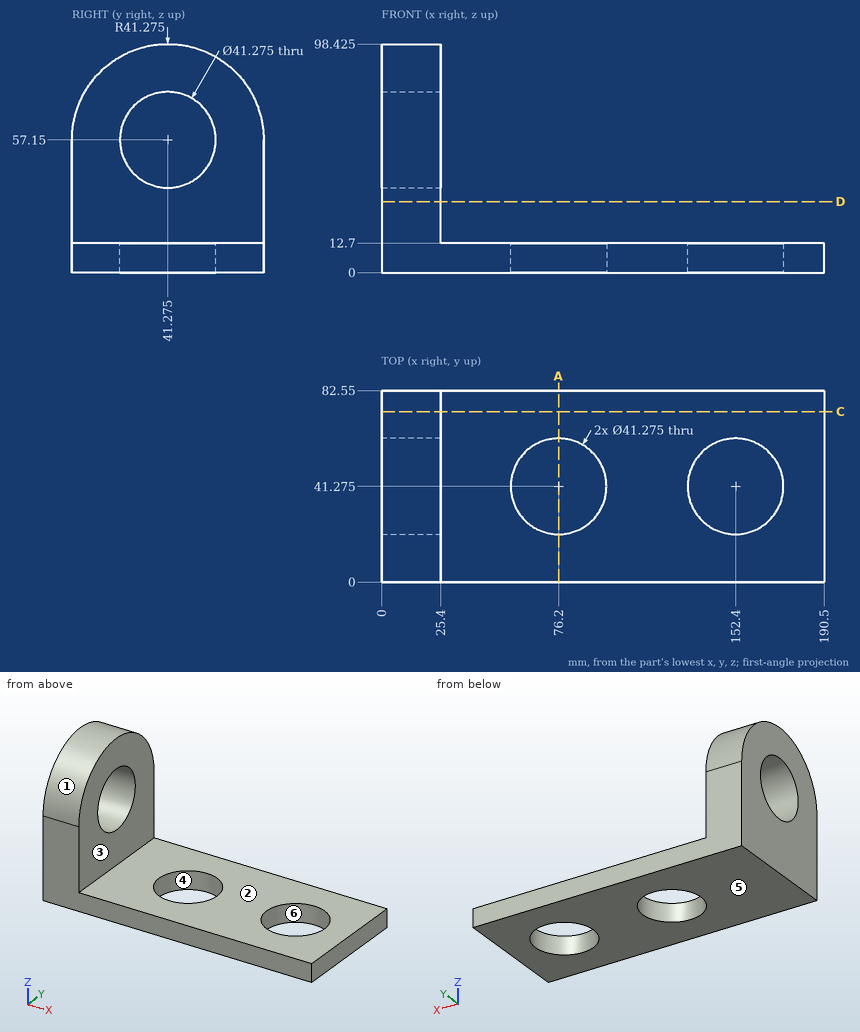
For this review, use the dimensioned drawing (mm, ordinates from the lowest corner) and the shaded views. A direction names the side the tool comes from. Round coordinates to 2 decimals unless told otherwise and drop trailing zeros. Order: outer loops, then holes, each group sorted by start corner. A loop starts at its lowest first (then second) coordinate and runs counter-clockwise, first axis right, second up. Notation, with made-up numbers: (-6, 67) -> (17, 67) arc R24 cw to (17, 90) -> close; hole circle Ø5 at (-4, 74.25). An arc over 180 degrees is marked (long way). Put each result on its own line as item: value.
Q1. Add section A-A on x = 76.2. Write out the cut boundary in (y, z).
Check result:
outline: (0, 0) -> (20.64, 0) -> (20.64, 12.7) -> (0, 12.7) -> close; (61.91, 0) -> (82.55, 0) -> (82.55, 12.7) -> (61.91, 12.7) -> close
Q2. Add section C-C on y = 73.5. Write out the cut boundary in (x, z), plus the area to 3 significant figures.
Check result:
outline: (0, 0) -> (190.5, 0) -> (190.5, 12.7) -> (25.4, 12.7) -> (25.4, 82.94) -> (0, 82.94) -> close
area: 4,200 mm2
Q3. Insertion check: pin 1 Ø4 at (y, z) = (34, 25.5) entering from +X. The pin has a flat end and moves straight along its axis. Give the tip position at first contact, or say it passes through.
Check result:
pin 1: x = 25.4
Q4. Mouldability with a two-part tool opening along X and no side actions: class the marked faces 3, 4, 5 and 6 as pulls with the +X half, pulls with the -X half, needs draft (parallel to the pull), parting line crosses it, or undercut.
Check result:
face 3: pulls with the +X half
face 4: undercut
face 5: needs draft
face 6: undercut
Q5. Machinability: for the marked faces 1 and 2, which of the approach directions +Z, -Z, +X, -X, +Y, -Y give a long, thin tool a straight path to every point of the face, cutting with its end or side? Answer none if there is none.
Check result:
face 1: +Z, +X, -X
face 2: +Z, +X, +Y, -Y
Q6. Add section D-D on z = 30.5. Write out the cut boundary in (x, y), plus the area to 3 significant figures.
Check result:
outline: (0, 0) -> (25.4, 0) -> (25.4, 82.55) -> (0, 82.55) -> close
area: 2,100 mm2
Q7. For probe 1 along Y at (x, z) = (152.4, 9.5); probe 2 along X at (y, z) = (49, 9); probe 3 along Z at (x, y) = (117.5, 72), list the stretches that pass through material, from the lowest coordinate up. Write a range as [from, to].
Check result:
probe 1: [0, 20.64], [61.91, 82.55]
probe 2: [0, 57.06], [95.34, 133.26], [171.54, 190.5]
probe 3: [0, 12.7]
